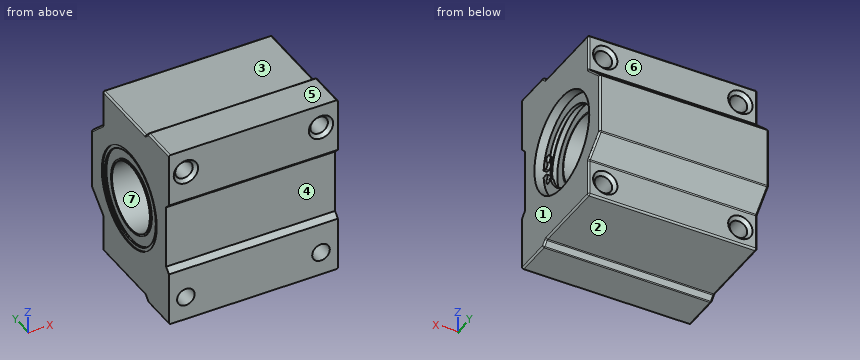
```python
from build123d import *

# Parameters (mm, degrees)
SKETCH1_R           = 14.5
BOSS_EXTRUDE1_DEPTH = 50
EXTRUDE_THIN1_START = 0.5
SKETCH1_4_R         = 10.5
SKETCH1_4_R_2       = 10
EXTRUDE_THIN1_DEPTH = 43.5
BOSS_EXTRUDE2_START = 0.8
SKETCH1_5_R         = 13.5
SKETCH1_5_R_2       = 10
BOSS_EXTRUDE2_DEPTH = 43
BOSS_EXTRUDE3_START = 0.3
SKETCH1_6_R         = 14.5
SKETCH1_6_R_2       = 13.5
BOSS_EXTRUDE3_DEPTH = 45
BOSS_EXTRUDE4_START = 1
BOSS_EXTRUDE4_DEPTH = 1
FILLET1_R           = 0.5
SKETCH4_R           = 2.6
CUT_EXTRUDE3_DEPTH  = 71.071392165
CHAMFER1_SIZE       = 1


with BuildPart() as part:
    # Sketch1 → Boss-Extrude1 (new body)
    with BuildSketch(Plane(origin=(0, 0, 0), x_dir=(0, 0, -1), z_dir=(1, 0, 0))):
        Polygon((-27, -10), (-25.5, -8.5), (-25.5, 14), (-14.5, 14), (-9, 20), (9, 20), (14.5, 14), (25.5, 14), (25.5, -8.5), (27, -10), (27, -21), (11, -21), (9.5, -19.5), (-9.5, -19.5), (-11, -21), (-27, -21), align=None)
        Circle(SKETCH1_R, mode=Mode.SUBTRACT)
    extrude(amount=BOSS_EXTRUDE1_DEPTH)



with BuildPart() as body_2:
    # Sketch1_4 → Extrude-Thin1 (new body)
    with BuildSketch(Plane(origin=(0, 0, 0), x_dir=(0, 0, -1), z_dir=(1, 0, 0)).offset(EXTRUDE_THIN1_START)):
        Circle(SKETCH1_4_R)
        Circle(SKETCH1_4_R_2, mode=Mode.SUBTRACT)
    extrude(amount=EXTRUDE_THIN1_DEPTH)

    # Sketch1_5 → Boss-Extrude2 (add)
    with BuildSketch(Plane(origin=(0, 0, 0), x_dir=(0, 0, -1), z_dir=(1, 0, 0)).offset(BOSS_EXTRUDE2_START)):
        Circle(SKETCH1_5_R)
        Circle(SKETCH1_5_R_2, mode=Mode.SUBTRACT)
    extrude(amount=BOSS_EXTRUDE2_DEPTH)


with BuildPart() as part_1:
    add(part.part)

    add(body_2.part)  # Boss-Extrude3 merges body 2
    # Sketch1_6 → Boss-Extrude3 (add)
    with BuildSketch(Plane(origin=(0, 0, 0), x_dir=(0, 0, -1), z_dir=(1, 0, 0)).offset(BOSS_EXTRUDE3_START)):
        Circle(SKETCH1_6_R)
        with Locations(Location((0, 0, 0), (0, 0, 180))):
            Circle(SKETCH1_6_R_2, mode=Mode.SUBTRACT)
    extrude(amount=BOSS_EXTRUDE3_DEPTH)

    # Sketch3 → Boss-Extrude4 (add)
    with BuildSketch(Plane(origin=(45.3, 0, 0), x_dir=(0, 0, -1), z_dir=(1, 0, 0)).offset(BOSS_EXTRUDE4_START)):
        with BuildLine():
            Line((-1.006226387, -13.462448086), (-1.080761675, -14.459666462))
            ThreePointArc((-1.080761675, -14.459666462), (0, 14.5), (1.080761675, -14.459666462))
            Line((1.080761675, -14.459666462), (1.006226387, -13.462448086))
            ThreePointArc((1.006226387, -13.462448086), (1.587963278, -12.439862683), (2.739999666, -12.678422687))
            ThreePointArc((2.739999666, -12.678422687), (4.399101385, -12.399835015), (3.456933265, -11.006081508))
            ThreePointArc((3.456933265, -11.006081508), (0, 11.53621332), (-3.456933265, -11.006081508))
            ThreePointArc((-3.456933265, -11.006081508), (-4.399101385, -12.399835015), (-2.739999666, -12.678422687))
            ThreePointArc((-2.739999666, -12.678422687), (-1.587963278, -12.439862683), (-1.006226387, -13.462448086))
        make_face()
    extrude(amount=BOSS_EXTRUDE4_DEPTH)

    # Fillet1
    fillet1_edges = [part_1.edges().sort_by_distance(p)[0] for p in [
        (50, -9.25, 26.25),
        (50, -15.5, 27),
        (0, 2.75, 25.5),
        (0, 14, 20),
        (0, 17, 11.75),
        (0, 20, 0),
        (0, 17, -11.75),
        (0, 14, -20),
        (0, 2.75, -25.5),
        (0, -9.25, -26.25),
        (0, -15.5, -27),
        (0, -15.5, 27),
        (0, -9.25, 26.25),
        (25, -8.5, 25.5),
        (25, 14, 25.5),
        (25, 14, 14.5),
        (25, 20, 9),
        (25, 20, -9),
        (25, 14, -14.5),
        (25, 14, -25.5),
        (25, -8.5, -25.5),
        (25, -10, -27),
        (25, -10, 27),
        (50, -15.5, -27),
        (50, -9.25, -26.25),
        (50, 2.75, -25.5),
        (50, 14, -20),
        (50, 17, -11.75),
        (50, 20, 0),
        (50, 17, 11.75),
        (50, 14, 20),
        (50, 2.75, 25.5),
    ]]
    fillet(fillet1_edges, radius=FILLET1_R)

    # Sketch4 → Cut-Extrude3 (cut, through all)
    with BuildSketch(Plane.XZ.offset(21)):
        with Locations(Location((5, 20, 0), (0, 0, 270))):
            Circle(SKETCH4_R)
        with Locations(Location((45, 20, 0), (0, 0, 270))):
            Circle(SKETCH4_R)
        with Locations(Location((45, -20, 0), (0, 0, 270))):
            Circle(SKETCH4_R)
        with Locations(Location((5, -20, 0), (0, 0, 270))):
            Circle(SKETCH4_R)
    extrude(amount=-CUT_EXTRUDE3_DEPTH, mode=Mode.SUBTRACT)

    # Chamfer1
    chamfer1_edges = [part_1.edges().sort_by_distance(p)[0] for p in [
        (5, 14, -17.4),
        (45, 14, -17.4),
        (45, 14, 22.6),
        (45, -21, 22.6),
        (5, 14, 22.6),
        (5, -21, 22.6),
    ]]
    chamfer(chamfer1_edges, length=CHAMFER1_SIZE)


solid = part_1.part
```
CAD build for the part. Positions are in the model's coordinates, mm. Face numbers are marked on the shaded views. A direction names the side the tool comes from. Coordinates: 2 decimals unless noted, no trailing zeros. Order: outer loops, then holes, each group sorted by start corner. A loop starts at its lowest first (then second) coordinate and runs counter-clockwise, first axis right, second up. Notation, with made-up numbers: (-5, 40) -> (28, 40) arc R26 ccw to (28, 54) -> close; hole circle Ø7 at (-33, 85.25). An arc over 180 degrees is marked (long way). Use one line per item in the form item = value. Start each with the question number.
1) Band-saw the part on C-C on y = 0. State how many separate pieces and enclosed holes the cut face has, then the cut area to 3 significant figures.
2) Drop flat-ended pins along their axis: pin 1 (11.5 mm diameter, centred on x = 29, z = -19.5, fed in from +Y); pin 2 (2 mm diameter, centred on x = 8.5, y = -6.5, fed in from +Z); pin 3 (10 mm diameter, centred on x = 12.5, y = 4, fed in from -Z). Give the stop position or say it passes through.
3) Band-saw the part on B-B on x = 21.5. Give the cut face in (y, z), then the cut area to 3 significant figures.
4) Tool access for the marked faces 1, 2, 3 and 4: list every direction of +Z, -Z, +X, -X, +Y, -Y with a clear straight run to the whole face (end or side of a thin tool).
5) Drill centre lines: L1, parallel to X at y = -8, z = 20; L2, parallel to Y at x = 22, z = 0; L3, parallel to Y at x = 4, z = 4. Where is each one in solid material? Low to high. Write a range as [from, to].
6) Band-saw the part on A-A on z = 20. Give the cut face in (x, y).
7) Pull direction Z, two halves, no side cores. Call the marked faces 5, 6 and 7: +Z half, -Z half, draft (parallel to the pull), parting line (faces both ways), or undercut.
Entries:
q1.separate_pieces = 2
q1.enclosed_holes = 4
q1.area = 1,410 mm2
q2.pin_1 = 14.82
q2.pin_2 = 25.5
q2.pin_3 = -25.5
q3.outline = (-21, -27) -> (-10.21, -27) arc R0.5 ccw to (-9.85, -26.85) -> (-8.65, -25.65) arc R0.5 cw to (-8.29, -25.5) -> (13.5, -25.5) arc R0.5 ccw to (14, -25) -> (14, -14.72) arc R0.5 cw to (14.16, -14.35) -> (19.84, -9.15) arc R0.5 ccw to (20, -8.78) -> (20, 8.78) arc R0.5 ccw to (19.84, 9.15) -> (14.16, 14.35) arc R0.5 cw to (14, 14.72) -> (14, 25) arc R0.5 ccw to (13.5, 25.5) -> (-8.29, 25.5) arc R0.5 cw to (-8.65, 25.65) -> (-9.85, 26.85) arc R0.5 ccw to (-10.21, 27) -> (-21, 27) -> (-21, 11) -> (-19.5, 9.5) -> (-19.5, -9.5) -> (-21, -11) -> close; hole circle Ø20 at (0, 0)
q3.area = 1,620 mm2
q4.face_1 = +Z, -Z, +X, +Y, -Y
q4.face_2 = -Z, +X, -X, +Y
q4.face_3 = +Z, +X, -X, +Y
q4.face_4 = +X, -X, -Y
q5.L1 = [0, 2.4], [7.6, 42.4], [47.6, 50]
q5.L2 = [-19.5, -10], [10, 20]
q5.L3 = [-19.5, -9.17], [9.17, 20]
q6.outline = (0, -21) -> (1.4, -21) -> (2.4, -20) -> (2.4, 13) -> (1.4, 14) -> (0.5, 14) arc R0.5 ccw to (0, 13.5) -> close; (7.6, -20) -> (8.6, -21) -> (41.4, -21) -> (42.4, -20) -> (42.4, 13) -> (41.4, 14) -> (8.6, 14) -> (7.6, 13) -> close; (47.6, -20) -> (48.6, -21) -> (50, -21) -> (50, 13.5) arc R0.5 ccw to (49.5, 14) -> (48.6, 14) -> (47.6, 13) -> close
q7.face_5 = +Z half
q7.face_6 = draft
q7.face_7 = undercut
